Autodesk Inventor part; units mm, degrees
ref_plane "YZ Plane" through (0, 0, 0) normal (1, 0, 0) x (0, 1, 0)
ref_plane "XZ Plane" through (0, 0, 0) normal (0, 1, 0) x (-1, 0, 0)
ref_plane "XY Plane" through (0, 0, 0) normal (0, 0, 1) x (1, 0, 0)
sketch "Boceto1" plane through (0, 0, 0) normal (0, 1, 0) x (-1, 0, 0)
  line L0 (105, 50) -> (-105, 50)
  line L1 (-105, 50) -> (-105, -50)
  line L2 (-105, -50) -> (105, -50)
  line L3 (105, -50) -> (105, 50)
  line L4 (105, 50) -> (-105, -50) construction
  line L5 (-105, 50) -> (105, -50) construction
  point P0 (0, 0)
  dimension "d0" = 210
  dimension "d1" = 100
extrude "Extrusión1" add sketch "Boceto1" along normal blind 20
sketch "Boceto2" plane through (0, 20, 0) normal (0, 1, 0) x (1, 0, 0)
  circle A0 centre (0, 3.5) radius 10
  circle A1 centre (31, -42.5) radius 3.5
  line L0 (0, 3.5) -> (21.5607, 3.5)
  circle A2 centre (31, 42.5) radius 3.5
  circle A3 centre (-28, 42.5) radius 3.5
  circle A4 centre (-28, -42.5) radius 3.5
  line L1 (105, 50) -> (-105, 50)
  point P0 (0, 0)
  dimension "d4" = 7
  dimension "d5" = 7
  dimension "d6" = 7
  dimension "d7" = 39
  dimension "d8" = 46
  dimension "d9" = 59
  dimension "d10" = 46
  dimension "d11" = 39
  dimension "d12" = 59
  dimension "d13" = 7.5
extrude "Extrusión2" cut sketch "Boceto2" against normal blind 20
sketch "Boceto3" plane through (0, 20, 0) normal (0, 1, 0) x (1, 0, 0)
  line L0 (-105, -50) -> (105, -50)
  line L1 (-45.0001, -10) -> (-45.0001, -50)
  line L2 (-75, -10) -> (-45.0001, -10)
  line L3 (-75, -50) -> (-75, -10)
  line L4 (-65, -50) -> (-75, -50)
  line L5 (-45.0001, -50) -> (-75, -50)
  line L6 (-55, -50.0503) -> (-45.0001, -50)
  line L7 (105, -50) -> (-105, -50)
  line L8 (55, -50.0503) -> (45.0001, -50)
  line L9 (65, -50) -> (75, -50)
  line L10 (-105, -50) -> (105, -50)
  line L11 (0, -50) -> (0, -28.25)
  line L12 (45.0001, -10) -> (45.0001, -50)
  line L13 (45.0001, -50) -> (75, -50)
  line L14 (75, -50) -> (75, -10)
  line L15 (75, -10) -> (45.0001, -10)
  point P0 (0, 0)
extrude "Extrusión3" cut sketch "Boceto3" against normal blind 10
sketch "Boceto4" plane through (-75, 20, 10) normal (0, 0, 1) x (1, 0, 0)
  line L0 (0, -10) -> (0, 0)
  line L1 (29.9999, -10) -> (0, -10)
  line L2 (0, 0) -> (29.9999, 0)
  line L3 (29.9999, 0) -> (29.9999, -10)
  line L4 (29.9999, -10) -> (0, -10)
  line L5 (0, -10) -> (0, 0)
  line L6 (120.0001, -10) -> (120.0001, 0)
  line L7 (150, -10) -> (120.0001, -10)
  line L8 (120.0001, 0) -> (150, 0)
  line L9 (150, 0) -> (150, -10)
  line L10 (150, -10) -> (120.0001, -10)
  line L11 (120.0001, -10) -> (120.0001, 0)
  point P0 (75, -20)
extrude "Extrusión4" add sketch "Boceto4" along normal blind 80
sketch "Boceto5" plane through (0, 20, 0) normal (0, 1, 0) x (1, 0, 0)
  circle A0 centre (56.75, -71.75) radius 1.75
  line L0 (55, -71.75) -> (55, -49.9497)
  circle A1 centre (63.25, -78.25) radius 1.75
  line L1 (65, -78.25) -> (65, -50)
  line L2 (55, -49.9497) -> (45.0001, -50)
  line L3 (65, -50) -> (75, -50)
  line L4 (45.0001, -50) -> (75, -50)
  line L5 (75, -50) -> (75, -90)
  line L6 (75, -90) -> (45.0001, -90)
  line L7 (45.0001, -90) -> (45.0001, -50)
  line L8 (0, -50) -> (0, -71.75)
  circle A2 centre (-56.75, -71.75) radius 1.75
  line L9 (-55, -71.75) -> (-55, -49.9497)
  circle A3 centre (-63.25, -78.25) radius 1.75
  line L10 (-65, -78.25) -> (-65, -50)
  line L11 (-45.0001, -50) -> (-75, -50)
  line L12 (-75, -50) -> (-75, -90)
  line L13 (-75, -90) -> (-45.0001, -90)
  line L14 (-45.0001, -90) -> (-45.0001, -50)
  line L15 (-45.0001, -90) -> (-75, -90)
  line L16 (-75, -50) -> (-75, -90)
  line L17 (-75, -20) -> (-51.4571, -20)
  line L18 (-45.0001, 50) -> (-45.0001, 10)
  line L19 (-45.0001, 10) -> (-15.0003, 10)
  line L20 (-35.0003, 31.75) -> (-35.0003, 9.9497)
  circle A4 centre (-33.2503, 31.75) radius 1.75
  line L21 (-25.0003, 38.25) -> (-25.0003, 10)
  circle A5 centre (-26.7503, 38.25) radius 1.75
  line L22 (-15.0003, 10) -> (-15.0003, 50)
  line L23 (-15.0003, 10) -> (-15.0003, 50)
  line L24 (-45.0001, 50) -> (-15.0003, 50)
  line L25 (-15.0003, 50) -> (-45.0001, 50)
  line L26 (-45.0001, 30) -> (-65.9082, 30)
  point P0 (0, 0)
  point P1 (105, 90)
  point P2 (105, 90)
  point P3 (63.25, -61.75)
  point P4 (56.75, -68.25)
  point P5 (-56.75, -68.25)
  point P6 (-63.25, -61.75)
  point P7 (105, 50)
  point P8 (-105, 50)
  point P9 (-33.2503, 28.25)
  point P10 (-26.7503, 21.75)
  dimension "d41" = 3.5
  dimension "d42" = 3.5
  dimension "d33" = 10
  dimension "d34" = 10
  dimension "d35" = 40
  dimension "d36" = 0
  dimension "d37" = 6.5
  dimension "d38" = 6.5
  dimension "d43" = 11.7499
  dimension "d44" = 11.75
hole "Agujero1" at (-56.75, 20, 71.75) at (-63.25, 20, 78.25) at (56.75, 20, 71.75) at (63.25, 20, 78.25) direction (0, -1, 0) diameter 3.5 end through all
sketch "Boceto6" plane through (105, 0, -50) normal (0, 0, -1) x (-1, 0, 0)
  line L0 (30, 20) -> (30, 10)
  line L1 (0, 0) -> (0, 20)
  line L2 (30, 20) -> (0, 20)
  line L3 (0, 20) -> (30, 20)
  line L4 (30, 20) -> (30, 10)
  line L5 (30, 10) -> (0, 10)
  line L6 (0, 10) -> (0, 20)
  line L7 (150.0001, 20) -> (59.9999, 20)
  line L8 (105, 20) -> (105, 8.0079)
  line L9 (180, 20) -> (180, 10)
  line L10 (210, 0) -> (210, 20)
  line L11 (180, 20) -> (210, 20)
  line L12 (210, 20) -> (180, 20)
  line L13 (180, 20) -> (180, 10)
  line L14 (180, 10) -> (210, 10)
  line L15 (210, 10) -> (210, 20)
  point P0 (105, 0)
  dimension "d70" = 30
  dimension "d71" = 30
extrude "Extrusión6" cut sketch "Boceto6" against normal blind 40
sketch "Boceto8" plane through (-105, 10, -50) normal (0, 1, 0) x (1, 0, 0)
  line L0 (0.0001, 0) -> (0.0001, -40)
  line L1 (30, -40) -> (30, 0)
  line L2 (-55.1959, 0.0503) -> (30, 0)
  line L3 (30, 0) -> (0.0001, 0)
  line L4 (0.0001, -40) -> (30, -40)
  line L5 (-64.3507, 0) -> (-74.3507, 0)
  circle A0 centre (18.2501, -28.25) radius 1.75
  circle A1 centre (11.7501, -21.75) radius 1.75
  line L6 (30, 0) -> (75.0001, 0)
  line L7 (180, 0) -> (30, 0)
  line L8 (30, 0) -> (30, -40)
  line L9 (210, 0) -> (0, 0)
  line L10 (105, 0) -> (105, -23.5)
  circle A2 centre (191.7499, -28.25) radius 1.75
  circle A3 centre (198.2499, -21.75) radius 1.75
  point P0 (105, -50)
  point P1 (18.2501, -21.75)
  point P2 (-63.4459, -118.25)
  point P3 (52.5001, 0)
  point P4 (191.7499, -21.75)
  dimension "d73" = 11.7499
  dimension "d74" = 40
  dimension "d75" = 29.9999
  dimension "d76" = 21.75
  dimension "d77" = 11.75
  dimension "d78" = 28.3003
  dimension "d79" = 11.7499
  dimension "d80" = 0
  dimension "d81" = 0
hole "Agujero3" at (-93.2499, 10, -28.25) at (-86.7499, 10, -21.75) at (86.7499, 10, -21.75) at (93.2499, 10, -28.25) direction (0, -1, 0) diameter 3.5 end through all
properties part number "base_mid"
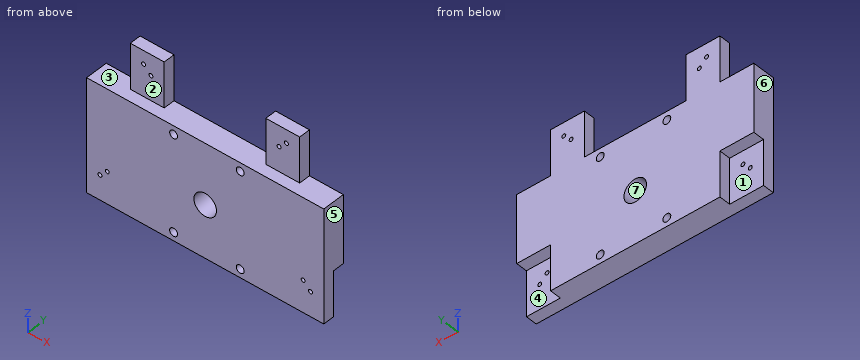
Source: CAD feature listing. Evaluate the final solid. Frame: model axes, mm. Face numbers are marked on the shaded views. A direction names the side the tool comes from. Give positions to 0.01 mm unless a question says otherwise; leave off trailing zeros. Loops run counter-clockwise (first coordinate to the right, second up) from the corner with the lowest first, then second, coordinate; pieces in that order, holes last. Notation, with made-up numbers: (22, -24) -> (70, -24) arc R33 cw to (70, 4) -> close; hole circle Ø4 at (-37, -20). An arc over 180 degrees is marked (long way). Put each result on its own line as item: value. Start each with the question number.
1) Contact query for flat-ended pins moving along their axis: P1, Ø15, axis at x = 95, z = -21, coming from the +Y side; P2, Ø4, axis at x = -63.25, z = 78.25, coming from the -Y side; P3, Ø3, axis at x = -58, y = 6.5, coming from the +Z side; P4, Ø16, axis at x = 0, z = -3.5, coming from the +Y side. Output: stop coordinate, or through.
2) Cut plane D-D (x = 3.5). Return loops of the section in (y, z).
3) Reachability of the marked faces 1, 2, 3 and 4 from +Z, -Z, +X, -X, +Y, -Y: full face, straight path, thin tool, end or side. Return the list, or none.
4) Draft query along X for the marked faces 5, 6 and 7. Return one class per face: released by +X, released by -X, zero draft, split by the parting line, or undercut.
5) Cut plane B-B (x = -28). Return loops of the section in (y, z).
6) Cut plane C-C (y = 12.25). State how many separate pieces and enclosed holes the cut face has, then the cut area to 3 significant figures.
7) Cut plane A-A (z = 42.5). Return loops of the section in (x, y), then the cut area to 3 significant figures.
8) Material intervals for probe 1 along Z at (x, y) = (-28, 7.5); probe 2 along X at (y, z) = (14.75, 71.75); probe 3 along X at (y, z) = (4.5, -21.75), sorted ascending.
Results are:
1. P1: stops at y = 10
1. P2: stops at y = 10
1. P3: stops at z = 50
1. P4: passes through
2. outline: (0, -50) -> (20, -50) -> (20, -12.87) -> (0, -12.87) -> close; (0, 5.87) -> (20, 5.87) -> (20, 50) -> (0, 50) -> close
3. face 1: -Z, -X, +Y
3. face 2: +Z, +X, -X, -Y
3. face 3: +Z, -Y
3. face 4: -Z, +X, +Y
4. face 5: released by +X
4. face 6: released by -X
4. face 7: undercut
5. outline: (0, -50) -> (20, -50) -> (20, -46) -> (0, -46) -> close; (0, -39) -> (20, -39) -> (20, 39) -> (0, 39) -> close; (0, 46) -> (20, 46) -> (20, 50) -> (0, 50) -> close
6. separate pieces: 1
6. enclosed holes: 9
6. area: 20,500 mm2
7. outline: (-105, 0) -> (-31.5, 0) -> (-31.5, 20) -> (-105, 20) -> close; (-24.5, 0) -> (27.5, 0) -> (27.5, 20) -> (-24.5, 20) -> close; (34.5, 0) -> (105, 0) -> (105, 20) -> (34.5, 20) -> close
7. area: 3,920 mm2
8. probe 1: z = -50 to -46, -39 to 39, 46 to 50
8. probe 2: x = -75 to -58.5, -55 to -45, 45 to 55, 58.5 to 75
8. probe 3: x = -105 to -88.5, -85 to 85, 88.5 to 105
